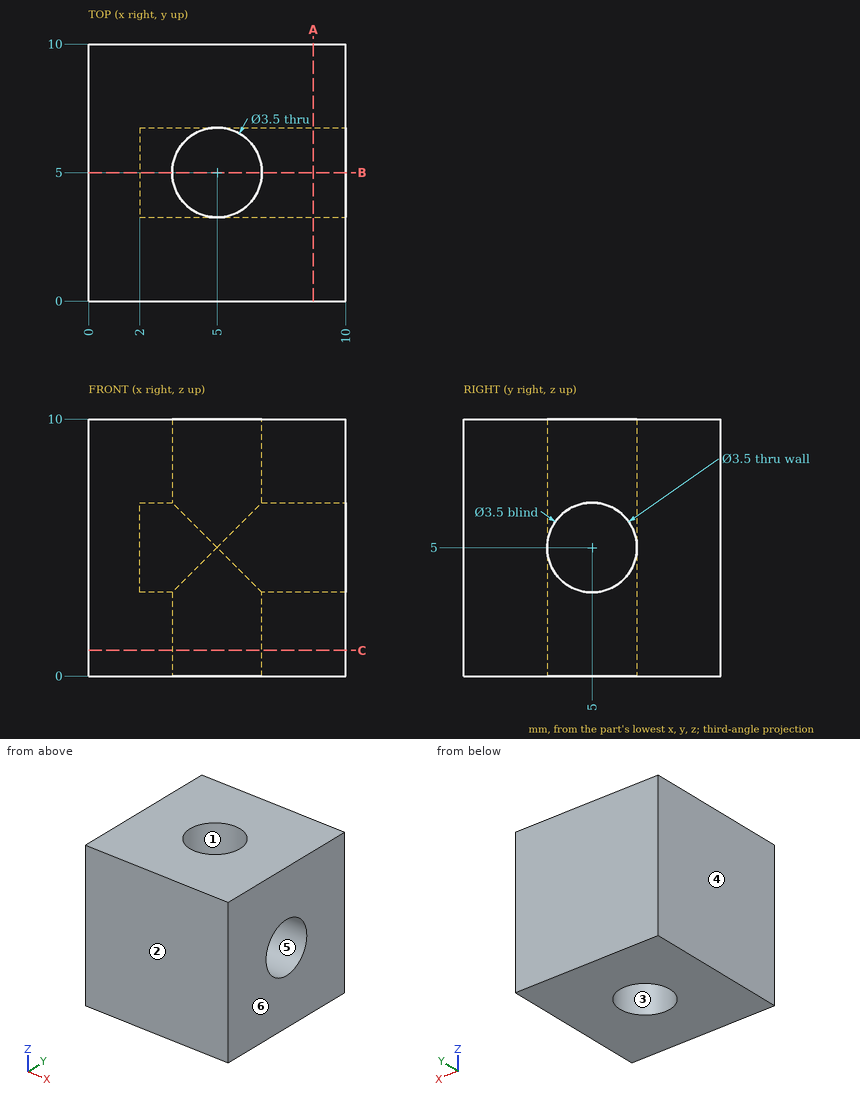
Check sheet for the drawn part. Datum: minimum x, y, z corner. Units: mm. A direction names the side the tool comes from. Round coordinates to 2 decimals unless told otherwise and drop trailing zeros. Order: outer loops, then holes, each group sorted by start corner. A loop starts at its lowest first (then second) coordinate and runs counter-clockwise, first axis right, second up. Notation, with made-up numbers: (18, 88.5) - (22, 88.5) arc R23 ccw to (22, 123.5) - close; hole circle Ø8 at (51.5, -37). An arc over 180 degrees is marked (long way). Use a Markdown table: item, result. Add a question column.
(1) Depth check by flat-ended pin: pin 1 (3 mm diameter, centred on y = 5, z = 5, fed in from +X). Enter the tip coordinate at first touch or a pass-through.
(2) Sectioned sample at A-A, the plane x = 8.75. Enter the section's corners in (y, z).
(3) Sectioned sample at B-B, the plane y = 5. Enter the section's corners in (x, z).
(4) Tool access check on the marked faces 5 and 6. Record the directions out of +Z, -Z, +X, -X, +Y, -Y that give a thin tool (end or side, any length) a straight path to the whole face; none if there is none.
(5) Release check for a two-part mould opening along Y. For the marked faces 1, 2, 3 and 4 record: pulls with the +Y half, pulls with the -Y half, needs draft (parallel to the pull), parting line crosses it, or undercut.
(6) Material ranges on line 1 along Y through (x, z) = (3.9, 5), recorded low to high. Write a range as [from, to].
Answers below:
| question | item | result |
|---|---|---|
| 1 | pin 1 | x = 2 |
| 2 | outline | (0, 0) - (10, 0) - (10, 10) - (0, 10) - close; hole circle Ø3.5 at (5, 5) |
| 3 | outline | (0, 0) - (3.25, 0) - (3.25, 3.25) - (2, 3.25) - (2, 6.75) - (3.25, 6.75) - (3.25, 10) - (0, 10) - close; (6.75, 0) - (10, 0) - (10, 3.25) - (6.75, 3.25) - close; (6.75, 6.75) - (10, 6.75) - (10, 10) - (6.75, 10) - close |
| 4 | face 5 | +X |
| 4 | face 6 | +Z, -Z, +X, +Y, -Y |
| 5 | face 1 | undercut |
| 5 | face 2 | pulls with the -Y half |
| 5 | face 3 | undercut |
| 5 | face 4 | needs draft |
| 6 | line 1 | [0, 3.25], [6.75, 10] |
